from build123d import *

# Parameters (mm, degrees)
SKETCH1_W           = 120
SKETCH1_H           = 120
BOSS_EXTRUDE1_DEPTH = 2
SKETCH2_R           = 1.775
CUT_EXTRUDE1_DEPTH  = 182.037166061
SKETCH3_R           = 1.775
CUT_EXTRUDE2_DEPTH  = 182.037166061


with BuildPart() as part:
    # Sketch1 → Boss-Extrude1 (new body)
    with BuildSketch(Plane(origin=(0, 0, 0), x_dir=(1, 0, 0), z_dir=(0, 1, 0))):
        with Locations((104.879995502, 14.733142437)):
            Rectangle(SKETCH1_W, SKETCH1_H)
    extrude(amount=BOSS_EXTRUDE1_DEPTH)

    # Sketch2 → Cut-Extrude1 (cut, through all)
    with BuildSketch(Plane(origin=(0, 2, 0), x_dir=(1, 0, 0), z_dir=(0, 1, 0))):
        with Locations(Location((65.379995502, 30.733142437, 0), (0, 0, 270))):
            Circle(SKETCH2_R)
        with Locations(Location((65.379995502, -1.266857563, 0), (0, 0, 270))):
            Circle(SKETCH2_R)
        with Locations(Location((144.379995502, -1.266857563, 0), (0, 0, 270))):
            Circle(SKETCH2_R)
        with Locations(Location((144.379995502, 30.733142437, 0), (0, 0, 270))):
            Circle(SKETCH2_R)
    extrude(amount=-CUT_EXTRUDE1_DEPTH, mode=Mode.SUBTRACT)

    # Sketch3 → Cut-Extrude2 (cut, through all)
    with BuildSketch(Plane(origin=(0, 2, 0), x_dir=(1, 0, 0), z_dir=(0, 1, 0))):
        with Locations(Location((79.379995502, -10.766857563, 0), (0, 0, 270))):
            Circle(SKETCH3_R)
        with Locations(Location((79.379995502, 40.233142437, 0), (0, 0, 270))):
            Circle(SKETCH3_R)
        with Locations(Location((130.379995502, -10.766857563, 0), (0, 0, 270))):
            Circle(SKETCH3_R)
        with Locations(Location((130.379995502, 40.233142437, 0), (0, 0, 270))):
            Circle(SKETCH3_R)
    extrude(amount=-CUT_EXTRUDE2_DEPTH, mode=Mode.SUBTRACT)


solid = part.part
The listing builds one solid part. Answer for the finished solid, in the listing's coordinates (mm). Coordinates: 2 decimals unless noted, no trailing zeros. Answer in a Markdown table with one row per item. Add a question column.
1. Determine the mould class of faces 1 (the flat face through (104, 2, -16)), 2 (the cylindrical face through (145.877, 1.014, -29.779)) for opening direction X: +X half, -X half, draft (parallel to the pull), parting line (faces both ways), or undercut.
2. Consider line 1 (X direction, y = 0.55, z = 10.5); line 2 (Z direction, x = 146, y = 1.8); line 3 (Z direction, x = 132, y = 0.25). Determine where each line is inside the solid, lowest interval first. Write a range as [from, to].
3. A flat-ended cylindrical pin translates along its axis: P1, Ø3, axis at x = 130.38, z = 10.77, coming from the +Y side. Find the tip coordinate at first contact, or state that the pin passes through.
Answer below:
| question | item | result |
|---|---|---|
| 1 | face 1 | draft |
| 1 | face 2 | undercut |
| 2 | line 1 | [44.88, 77.63], [81.13, 128.63], [132.13, 164.88] |
| 2 | line 2 | [-74.73, -31.46], [-30.01, 0.54], [1.99, 45.27] |
| 2 | line 3 | [-74.73, -40.96], [-39.51, 10.04], [11.49, 45.27] |
| 3 | P1 | through |
